```python
from build123d import *

# Parameters (mm, degrees)
BOSS_EXTRUDE1_DEPTH = 2.93
SKETCH2_R           = 5
BOSS_EXTRUDE2_DEPTH = 4.7
CUT_EXTRUDE1_REACH  = 34.806
SKETCH3_R           = 2.75
CUT_EXTRUDE2_REACH  = 34.251
SKETCH4_R           = 1.5


with BuildPart() as part:
    # Sketch1 → Boss-Extrude1 (new body)
    with BuildSketch(Plane(origin=(0, 0, 0), x_dir=(1, 0, 0), z_dir=(0, 1, 0))):
        with BuildLine():
            Line((-5.5, 0), (-6.26, 0))
            ThreePointArc((-6.26, 0), (-10.149087297, -1.610912703), (-11.76, -5.5))
            Line((-11.76, -5.5), (-11.76, -24.16))
            ThreePointArc((-11.76, -24.16), (-10.149087297, -28.049087297), (-6.26, -29.66))
            Line((-6.26, -29.66), (-5.5, -29.66))
            ThreePointArc((-5.5, -29.66), (-1.610912703, -28.049087297), (0, -24.16))
            Line((0, -24.16), (0, -5.5))
            ThreePointArc((0, -5.5), (-1.610912703, -1.610912703), (-5.5, 0))
        make_face()
    extrude(amount=BOSS_EXTRUDE1_DEPTH)

    # Sketch2 → Boss-Extrude2 (add)
    with BuildSketch(Plane(origin=(0, 2.93, 0), x_dir=(1, 0, 0), z_dir=(0, 1, 0))):
        with Locations(Location((-5.88, -23.93, 0), (0, 0, 270))):
            Circle(SKETCH2_R)
    extrude(amount=BOSS_EXTRUDE2_DEPTH)

    # Sketch3 → Cut-Extrude1 (cut, up to next)
    with BuildSketch(Plane(origin=(0, 7.63, 0), x_dir=(1, 0, 0), z_dir=(0, 1, 0)), mode=Mode.PRIVATE) as cut_extrude1_sk1:
        with Locations(Location((-5.88, -23.93, 0), (0, 0, 270))):
            Circle(SKETCH3_R)
    cut_extrude1_tool1 = extrude(cut_extrude1_sk1.sketch, amount=-CUT_EXTRUDE1_REACH, mode=Mode.PRIVATE) & part.part
    add(cut_extrude1_tool1.solids().sort_by_distance((-5.88, 7.63, 23.93))[0], mode=Mode.SUBTRACT)

    # Sketch4 → Cut-Extrude2 (cut, up to next)
    with BuildSketch(Plane(origin=(0, 2.93, 0), x_dir=(1, 0, 0), z_dir=(0, 1, 0)), mode=Mode.PRIVATE) as cut_extrude2_sk1:
        with Locations(Location((-5.88, -4, 0), (0, 0, 270))):
            Circle(SKETCH4_R)
    cut_extrude2_tool1 = extrude(cut_extrude2_sk1.sketch, amount=-CUT_EXTRUDE2_REACH, mode=Mode.PRIVATE) & part.part
    # Sketch4 → Cut-Extrude2 (cut, up to next)
    with BuildSketch(Plane(origin=(0, 2.93, 0), x_dir=(1, 0, 0), z_dir=(0, 1, 0)), mode=Mode.PRIVATE) as cut_extrude2_sk2:
        with Locations(Location((-5.88, -9.8, 0), (0, 0, 270))):
            Circle(SKETCH4_R)
    cut_extrude2_tool2 = extrude(cut_extrude2_sk2.sketch, amount=-CUT_EXTRUDE2_REACH, mode=Mode.PRIVATE) & part.part
    add(cut_extrude2_tool1.solids().sort_by_distance((-5.88, 2.93, 4))[0], mode=Mode.SUBTRACT)
    add(cut_extrude2_tool2.solids().sort_by_distance((-5.88, 2.93, 9.8))[0], mode=Mode.SUBTRACT)


solid = part.part
```
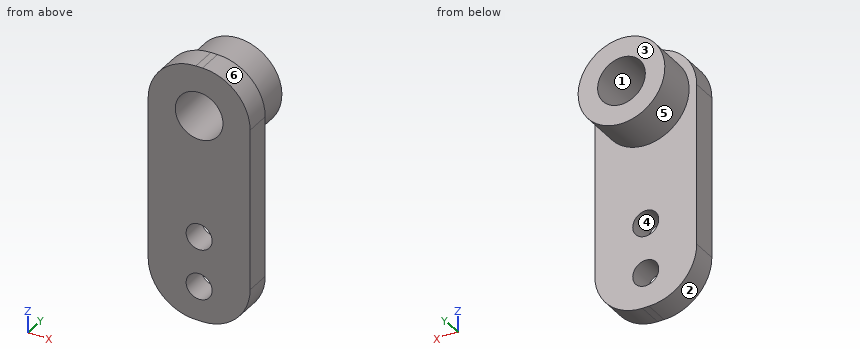
Read the model definition and answer for the solid it produces. Units are mm, in the model's axes. Face numbers are marked on the shaded views. A direction names the side the tool comes from. Round coordinates to 2 decimals unless told otherwise and drop trailing zeros. Write each loop counter-clockwise with the first axis right and the second up, starting at its lowest first coordinate (ties: lowest second). Pieces come first, ordered by that corner, then holes. Notation, with made-up numbers: M -14.75,44 L 28.25,44 A23 ccw 28.25,61 Z; hole C 13,87.5 d7. An arc over 180 degrees is marked long. One line per item, written item: value.
Q1. Find section A-A on x = -5.88. Write down the section's boundary in (y, z), plus the area to 3 significant figures.
Data:
outline: M 0,0 L 2.93,0 L 2.93,2.5 L 0,2.5 Z; M 0,5.5 L 2.93,5.5 L 2.93,8.3 L 0,8.3 Z; M 0,11.3 L 2.93,11.3 L 2.93,18.93 L 7.63,18.93 L 7.63,21.18 L 0,21.18 Z; M 0,26.68 L 7.63,26.68 L 7.63,28.93 L 2.93,28.93 L 2.93,29.66 L 0,29.66 Z
area: 74.4 mm2
Q2. Straight lines are drawn through the part: line 1 (Z direction, x = -5.25, y = 2); line 2 (Y direction, x = -4.5, z = 10.75); line 3 (X direction, y = 0.95, z = 9.8). For each, find the intervals that lie inside material, in ascending order. Write a range as [from, to].
Data:
line 1: [0.01, 2.64], [5.36, 8.44], [11.16, 21.25], [26.61, 29.65]
line 2: [0, 2.93]
line 3: [-11.76, -7.38], [-4.38, 0]
Q3. Find section D-D on y = 5.25. Write down the section's boundary in (x, z), plus the area to 3 significant figures.
Data:
outline: C -5.88,23.93 d10; hole C -5.88,23.93 d5.5
area: 54.8 mm2
Q4. Find section C-C on x = -9.75. Write down the section's boundary in (y, z), plus the area to 3 significant figures.
Data:
outline: M 0,1.25 L 2.93,1.25 L 2.93,20.76 L 7.63,20.76 L 7.63,27.1 L 2.93,27.1 L 2.93,28.41 L 0,28.41 Z
area: 109 mm2
Q5. Flat-ended cylindrical pins translate along their axes: pin 1 Ø3.5 at (x, z) = (-5.88, 9.8) entering from +Y; pin 2 Ø3 at (y, z) = (3, 21.5) entering from -X; pin 3 Ø2 at (x, y) = (-5.5, 5) entering from +Z. Find the tip coordinate at first contact, or state that the pin passes through.
Data:
pin 1: y = 2.93
pin 2: x = -11.76
pin 3: z = 28.93
Q6. For a pull along X with two mould halves and no side action, classify the marked faces 1, 2, 3 and 4 as +X half, -X half, draft (parallel to the pull), parting line (faces both ways), or undercut.
Data:
face 1: undercut
face 2: -X half
face 3: draft
face 4: undercut
Q7. Find section B-B on z = 9. Write down the section's boundary in (x, y), plus the area to 3 significant figures.
Data:
outline: M -11.76,0 L -7.15,0 L -7.15,2.93 L -11.76,2.93 Z; M -4.61,0 L 0,0 L 0,2.93 L -4.61,2.93 Z
area: 27.0 mm2
Q8. Which of the six approach directions +Z, -Z, +X, -X, +Y, -Y give full straight-line access (tool end or side, diameter ignored) to the marked faces 5 and 6?
Data:
face 5: +Y
face 6: +Z, +X, +Y, -Y
